Source: CAD feature listing. Evaluate the final solid. Frame: model axes, mm. A direction names the side the tool comes from. Give positions to 0.01 mm unless a question says otherwise; leave off trailing zeros. Write each loop counter-clockwise with the first axis right and the second up, starting at its lowest first coordinate (ties: lowest second). Pieces come first, ordered by that corner, then holes.
```python
from build123d import *

# Parameters (mm, degrees)
SKETCH1_W                   = 68.548183611
SKETCH1_H                   = 64.912098736
BOSS_EXTRUDE1_DEPTH         = 3.175
F_1_4_0_25_DIAMETER_HOLE1_D = 6.35
CUT_EXTRUDE1_DEPTH          = 95.459063428
FILLET1_R                   = 6.604
SKETCH5_W                   = 3.175
SKETCH5_H                   = 12.7
BOSS_EXTRUDE2_DEPTH         = 3.175


with BuildPart() as part:
    # Sketch1 → Boss-Extrude1 (new body)
    with BuildSketch(Plane.XY):
        with Locations((34.274091805, 32.456049368)):
            Rectangle(SKETCH1_W, SKETCH1_H)
    extrude(amount=BOSS_EXTRUDE1_DEPTH)

    # 1/4 (0.25) Diameter Hole1 (through all)
    with Locations(Plane(origin=(0, 0, 0), x_dir=(-1, 0, 0), z_dir=(0, 0, -1))):
        with Locations((-18.542, 44.846098736)):
            Hole(F_1_4_0_25_DIAMETER_HOLE1_D / 2)

    # Sketch4 → Cut-Extrude1 (cut, through all)
    with BuildSketch(Plane(origin=(0, 0, 0), x_dir=(-1, 0, 0), z_dir=(0, 0, -1))):
        Polygon((-26.0096, 48.402098736), (0, 64.912098736), (-68.548183611, 64.912098736), (-68.548183611, 0), (0, 0), (0, 33.293092607), (-26.0096, 39.512098736), align=None)
    extrude(amount=-CUT_EXTRUDE1_DEPTH, mode=Mode.SUBTRACT)

    # Fillet1
    fillet1_edges = [part.edges().sort_by_distance(p)[0] for p in [
        (26.0096, 39.512098736, 1.5875),
        (26.0096, 48.402098736, 1.5875),
    ]]
    fillet(fillet1_edges, radius=FILLET1_R)

    # Sketch5 → Boss-Extrude2 (add)
    with BuildSketch(Plane(origin=(0, 0, 0), x_dir=(-1, 0, 0), z_dir=(0, 0, -1))):
        with Locations((1.5875, 48.533092607)):
            Rectangle(SKETCH5_W, SKETCH5_H)
    extrude(amount=-BOSS_EXTRUDE2_DEPTH)


solid = part.part
```
1. Access query for faces 1 (the flat face through (11.63, 57.53, 1.57)), 2 (the flat face through (-2, 42.183, 2)), 3 (the flat face through (-2, 54.883, 2)). Directions: +Z, -Z, +X, -X, +Y, -Y. A direction counts if a zero-diameter tool reaches every point of the face in a straight line with its end or side. Return the directions, or none.
2. Line query: probe 1 along Y at (x, z) = (-0.5, 0.45); probe 2 along Y at (x, z) = (17.75, 2.4) (3 decimals); probe 3 along X at (y, z) = (46.5, 1.75) (1 decimal). Output: solid intervals per line, ascending.
3. Section query A-A (x = 18). Return loops of the section in (y, z) (1 decimal).
4. Section query C-C (z = 1). Return loops of the section in (x, y) (3 decimals), plus the area to 3 significant figures.
5. Section query D-D (x = -1.5). Return loops of the section in (y, z) (3 decimals).
6. Section query B-B (y = 44). Return loops of the section in (x, z) (3 decimals), plus the area to 3 significant figures.
7. Pin query (flat end, axial travel): P1, Ø1, axis at x = -2, z = 1.5, coming from the -Y side; P2, Ø1.5, axis at x = 19, z = 2.5, coming from the +Y side; P3, Ø1, axis at y = 57.5, z = 1, coming from the -X side. Return the tip coordinate at first contact, or that it passes through.
8. Pull-direction query (X, two-part tool) for faces 4 (the flat face through (-3.175, 48, 2)), 5 (the cylindrical face through (17.854, 41.747, 1.61)), 6 (the cylindrical face through (24.55, 40.58, 1.61)), 7 (the flat face through (8, 46, 0)); classes: pulls with the +X half, pulls with the -X half, needs draft (parallel to the pull), parting line crosses it, or undercut.
The answers:
1. face 1: +Z, -Z, +X, +Y
1. face 2: +Z, -Z, -X, -Y
1. face 3: +Z, -Z, -X, +Y
2. probe 1: y = 42.18 to 54.88
2. probe 2: y = 37.537 to 41.771, 47.921 to 53.645
2. probe 3: x = -3.2 to 15.8, 21.3 to 25.8
3. outline: (37.6, 0) - (41.7, 0) - (41.7, 3.2) - (37.6, 3.2) - close; (48, 0) - (53.5, 0) - (53.5, 3.2) - (48, 3.2) - close
4. outline: (-3.175, 42.183) - (0, 42.183) - (0, 33.293) - (20.941, 38.3) arc R6.604 ccw to (26.01, 44.723) - (26.01, 44.772) arc R6.604 ccw to (22.945, 50.348) - (0, 64.912) - (0, 54.883) - (-3.175, 54.883) - close; hole circle Ø6.35 at (18.542, 44.846)
4. area: 528 mm2
5. outline: (42.183, 0) - (54.883, 0) - (54.883, 3.175) - (42.183, 3.175) - close
6. outline: (-3.175, 0) - (15.482, 0) - (15.482, 3.175) - (-3.175, 3.175) - close; (21.602, 0) - (25.97, 0) - (25.97, 3.175) - (21.602, 3.175) - close
6. area: 73.1 mm2
7. P1: stops at y = 42.18
7. P2: stops at y = 53.33
7. P3: stops at x = 0
8. face 4: pulls with the -X half
8. face 5: undercut
8. face 6: pulls with the +X half
8. face 7: needs draft
